Here's how the part is built. I have some questions about the finished solid (model axes, mm). Give positions to 0.01 mm unless a question says otherwise; leave off trailing zeros. Order: outer loops, then holes, each group sorted by start corner. A loop starts at its lowest first (then second) coordinate and runs counter-clockwise, first axis right, second up. Notation, with made-up numbers: (3, -32.75) - (40, -32.75) arc R21 cw to (40, -16.75) - close; hole circle Ø3 at (60.5, 46). An arc over 180 degrees is marked (long way). One line per question, with ' | ' between items.
from build123d import *

# Parameters (mm, degrees)
F1_DEPTH  = 8
F3_W      = 8
F3_H      = 8
F3_R      = 2.4
F4_DEPTH  = 1.7
F5_R      = 2.4
F6_DEPTH  = 1.7
F14_W     = 25.3485813737
F14_H     = 15.2238979936
F15_DEPTH = 48.006


with BuildPart() as f1:
    # F0 (on Front) → F1 (new body)
    with BuildSketch(Plane.XZ):
        Polygon((-2.4, 3.2333333013), (-4, 3.2333333013), (-4, 0), (4, 0), (4, 3.2333333013), (2.4, 3.2333333013), (2.4, 4.9333333013), (-2.4, 4.9333333013), align=None)
    extrude(amount=F1_DEPTH)

    # F3 (on plane+point) → F4 (cut, through all)
    with BuildSketch(Plane.XY.offset(4.9333333013)):
        with Locations((0, -4)):
            Rectangle(F3_W, F3_H)
        with Locations((0, -4)):
            Circle(F3_R, mode=Mode.SUBTRACT)
    extrude(amount=-F4_DEPTH, mode=Mode.SUBTRACT)

    # F5 (on Top) → F6 (cut)
    with BuildSketch(Plane.XY):
        with Locations((0, -4)):
            Circle(F5_R)
    extrude(amount=F6_DEPTH, mode=Mode.SUBTRACT)

    # F8: F1 across plane


with BuildPart() as f1_1:
    add(f1.part)
    add(f1.part.mirror(Plane.YZ.offset(4)))

    # F9: F1 across plane


with BuildPart() as f1_2:
    add(f1_1.part)
    add(f1_1.part.mirror(Plane.XZ))

    # F11: F1 across plane


with BuildPart() as f1_3:
    add(f1_2.part)
    add(f1_2.part.mirror(Plane.YZ.offset(12)))

    # F12: F1 across face


with BuildPart() as f1_4:
    add(f1_3.part)
    add(f1_3.part.mirror(Plane(origin=(28, 0, 1.6166666507), x_dir=(0, 1, 0), z_dir=(1, 0, 0))))

    # F13: F1 across face


with BuildPart() as f1_5:
    add(f1_4.part)
    add(f1_4.part.mirror(Plane(origin=(60, 0, 1.6166666507), x_dir=(0, 1, 0), z_dir=(1, 0, 0))))

    # F14 (on face) → F15 (cut)
    with BuildSketch(Plane.YZ.offset(124)):
        with Locations((4.5101642609, 0)):
            Rectangle(F14_W, F14_H)
    extrude(amount=-F15_DEPTH, mode=Mode.SUBTRACT)


solid = f1_5.part
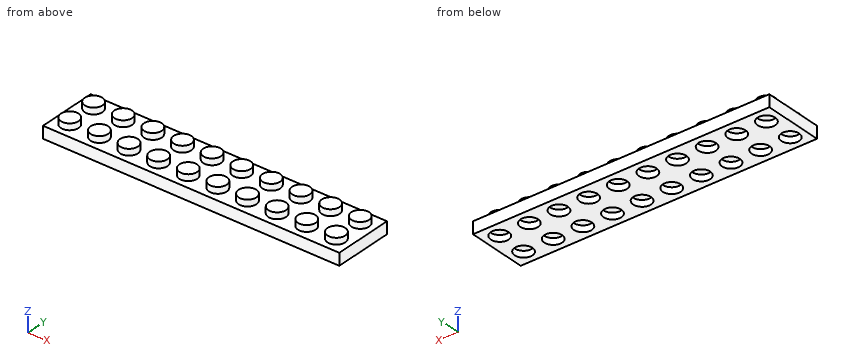
1) I want a section at A-A (x = 22.5). List the corners of the cut face in (y, z) for me, plus the area to 3 significant figures.
Model answer:
outline: (-8, 0) - (-5.87, 0) - (-5.87, 1.7) - (-2.13, 1.7) - (-2.13, 0) - (2.13, 0) - (2.13, 1.7) - (5.87, 1.7) - (5.87, 0) - (8, 0) - (8, 3.23) - (5.87, 3.23) - (5.87, 4.93) - (2.13, 4.93) - (2.13, 3.23) - (-2.13, 3.23) - (-2.13, 4.93) - (-5.87, 4.93) - (-5.87, 3.23) - (-8, 3.23) - close | area: 51.7 mm2
2) I'm going to push flat-ended pins straight in: P1, Ø4.5, axis at x = 8, y = 4, coming from the -Z side; P2, Ø1.5, axis at y = 2.5, z = 4.5, coming from the +X side; P3, Ø1, axis at y = 6, z = 4.5, coming from the +X side. Where does each tip first touch, or does it pass through?
Model answer:
P1: stops at z = 1.7 | P2: stops at x = 74.28 | P3: stops at x = 73.87
3) Please list where these lines run through material, in increasing order: L1, parallel to Y at x = 0, z = 1.15; L2, parallel to Z at x = 41, y = 2.5; L3, parallel to Z at x = 69.5, y = 5.5.
Model answer:
L1: y = -8 to -6.4, -1.6 to 1.6, 6.4 to 8 | L2: z = 1.7 to 4.93 | L3: z = 0 to 3.23
4) I want a section at B-B (y = -0.25). List the corners of the cut face in (x, z) for me, plus the area to 3 significant figures.
Model answer:
outline: (-4, 0) - (75.99, 0) - (75.99, 3.23) - (-4, 3.23) - close | area: 259 mm2
